For this review, take the finished solid that the model builds, in its own axes (mm). Face numbers are marked on the shaded views. A direction names the side the tool comes from. Round coordinates to 2 decimals unless told otherwise and drop trailing zeros. Write each loop counter-clockwise with the first axis right and the second up, starting at its lowest first coordinate (ties: lowest second). Pieces come first, ordered by that corner, then holes. Notation, with made-up numbers: (60, -24) -> (74, -24) arc R27 ccw to (74, 9) -> close; hole circle Ø8 at (73, -15.5). An arc over 180 degrees is marked (long way). Answer in a Markdown table with one row per item.
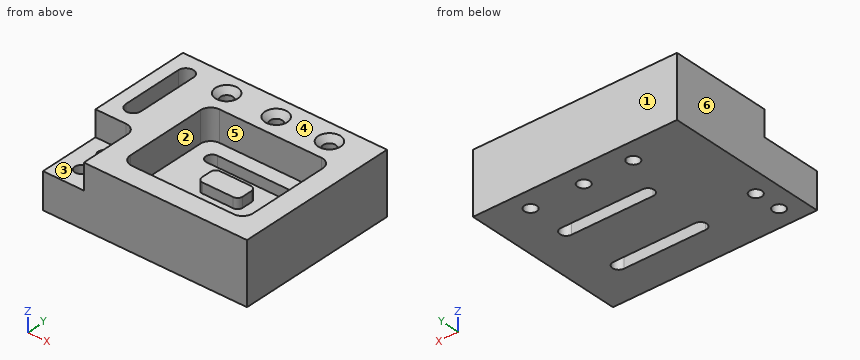
from build123d import *

# Parameters (mm, degrees)
SKETCH1_W           = 200
SKETCH1_H           = 160
BASE_EXTRUDE_DEPTH  = 60
CUT_EXTRUDE1_DEPTH  = 30
CUT_EXTRUDE2_DEPTH  = 25
HOLE1_D             = 12
HOLE1_CSINK_D       = 22
HOLE1_CSINK_ANGLE   = 82
HOLE4_D             = 12
HOLE4_CSINK_D       = 22
HOLE4_CSINK_ANGLE   = 82
HOLE5_D             = 12
HOLE5_CSINK_D       = 22
HOLE5_CSINK_ANGLE   = 82
SKETCH21_R          = 6
CUT_EXTRUDE4_DEPTH  = 133.759180474
CUT_EXTRUDE5_DEPTH  = 25
CUT_EXTRUDE6_DEPTH  = 132.52946438
BOSS_EXTRUDE1_DEPTH = 10


with BuildPart() as part:
    # Sketch1 → Base-Extrude (new body)
    with BuildSketch(Plane.XY):
        Rectangle(SKETCH1_W, SKETCH1_H)
    extrude(amount=-BASE_EXTRUDE_DEPTH)

    # Sketch2 → Cut-Extrude1 (cut)
    with BuildSketch(Plane.XY):
        with BuildLine():
            Line((-30, 40), (70, 40))
            ThreePointArc((70, 40), (77.071067812, 37.071067812), (80, 30))
            Line((80, 30), (80, -50))
            ThreePointArc((80, -50), (77.071067812, -57.071067812), (70, -60))
            Line((70, -60), (-30, -60))
            ThreePointArc((-30, -60), (-37.071067812, -57.071067812), (-40, -50))
            Line((-40, -50), (-40, 30))
            ThreePointArc((-40, 30), (-37.071067812, 37.071067812), (-30, 40))
        make_face()
    extrude(amount=-CUT_EXTRUDE1_DEPTH, mode=Mode.SUBTRACT)

    # Sketch3 → Cut-Extrude2 (cut)
    with BuildSketch(Plane.XY):
        with BuildLine():
            Line((-120, -20), (-70, -20))
            ThreePointArc((-70, -20), (-62.928932188, -22.928932188), (-60, -30))
            Line((-60, -30), (-60, -100))
            Line((-60, -100), (-120, -100))
            Line((-120, -100), (-120, -20))
        make_face()
    extrude(amount=-CUT_EXTRUDE2_DEPTH, mode=Mode.SUBTRACT)

    # Hole1 (through all)
    with Locations(Plane.XY):
        with Locations((-40, 60)):
            CounterSinkHole(HOLE1_D / 2, HOLE1_CSINK_D / 2, counter_sink_angle=HOLE1_CSINK_ANGLE)

    # Hole4 (through all)
    with Locations(Plane(origin=(41.997272993, -0.127725249, 0), x_dir=(1, 0, 0), z_dir=(0, 0, 1))):
        with Locations((-33.333333333, 60)):
            CounterSinkHole(HOLE4_D / 2, HOLE4_CSINK_D / 2, counter_sink_angle=HOLE4_CSINK_ANGLE)

    # Hole5 (through all)
    with Locations(Plane(origin=(100.148393301, 0.657149803, 0), x_dir=(1, 0, 0), z_dir=(0, 0, 1))):
        with Locations((-40, 60)):
            CounterSinkHole(HOLE5_D / 2, HOLE5_CSINK_D / 2, counter_sink_angle=HOLE5_CSINK_ANGLE)

    # Sketch21 → Cut-Extrude4 (cut, through all)
    with BuildSketch(Plane.XY.offset(-25)):
        with Locations((-80, -33.333333333)):
            Circle(SKETCH21_R)
        with Locations((-80, -60)):
            Circle(SKETCH21_R)
    extrude(amount=-CUT_EXTRUDE4_DEPTH, mode=Mode.SUBTRACT)

    # Sketch22 → Cut-Extrude5 (cut)
    with BuildSketch(Plane.XY):
        with BuildLine():
            Line((-72.5, 60), (-72.5, 0))
            ThreePointArc((-72.5, 0), (-80, -7.5), (-87.5, 0))
            Line((-87.5, 0), (-87.5, 60))
            ThreePointArc((-87.5, 60), (-80, 67.5), (-72.5, 60))
        make_face()
    extrude(amount=-CUT_EXTRUDE5_DEPTH, mode=Mode.SUBTRACT)

    # Sketch23 → Cut-Extrude6 (cut, through all)
    with BuildSketch(Plane.XY.offset(-30)):
        with BuildLine():
            Line((-20, 26), (60.148393301, 26))
            ThreePointArc((60.148393301, 26), (66.148393301, 20), (60.148393301, 14))
            Line((60.148393301, 14), (-20, 14))
            ThreePointArc((-20, 14), (-26, 20), (-20, 26))
        make_face()
        with BuildLine():
            Line((-20, -34), (60.148393301, -34))
            ThreePointArc((60.148393301, -34), (66.148393301, -40), (60.148393301, -46))
            Line((60.148393301, -46), (-20, -46))
            ThreePointArc((-20, -46), (-26, -40), (-20, -34))
        make_face()
    extrude(amount=-CUT_EXTRUDE6_DEPTH, mode=Mode.SUBTRACT)

    # Sketch24 → Boss-Extrude1 (add)
    with BuildSketch(Plane.XY.offset(-30)):
        with BuildLine():
            Line((5, 0), (35, 0))
            ThreePointArc((35, 0), (38.535533906, -1.464466094), (40, -5))
            Line((40, -5), (40, -15))
            ThreePointArc((40, -15), (38.535533906, -18.535533906), (35, -20))
            Line((35, -20), (5, -20))
            ThreePointArc((5, -20), (1.464466094, -18.535533906), (0, -15))
            Line((0, -15), (0, -5))
            ThreePointArc((0, -5), (1.464466094, -1.464466094), (5, 0))
        make_face()
    extrude(amount=BOSS_EXTRUDE1_DEPTH)


solid = part.part
1) Clearance check with flat-ended pins moving along their axes: pin 1 Ø1.5 at (x, y) = (36.5, -11) entering from +Z; pin 2 Ø4.5 at (x, y) = (-79, 19.5) entering from +Z. State where each tip first meets the part, or that it passes through.
Solved:
| item | result |
|---|---|
| pin 1 | z = -20 |
| pin 2 | z = -25 |
2) Consider section C-C on z = -46. State the section outline as (x, y) points, then the cut area to 3 significant figures.
Solved:
| item | result |
|---|---|
| outline | (-100, -80) -> (100, -80) -> (100, 80) -> (-100, 80) -> close; hole circle Ø12 at (-80, -60); hole circle Ø12 at (-80, -33.33); hole circle Ø12 at (-40, 60); hole (-20, -46) -> (60.15, -46) arc R6 ccw to (60.15, -34) -> (-20, -34) arc R6 ccw to start; hole (-20, 14) -> (60.15, 14) arc R6 ccw to (60.15, 26) -> (-20, 26) arc R6 ccw to start; hole circle Ø12 at (8.66, 59.87); hole circle Ø12 at (60.15, 60.66) |
| area | 29,300 mm² |
3) For line 1 (Y direction, x = -80, z = -51); line 2 (Y direction, x = -12.5, z = -41.5); line 3 (X direction, y = 60, z = -47), list the stretches that pass through material, from the lowest coordinate up. Write a range as [from, to].
Solved:
| item | result |
|---|---|
| line 1 | [-80, -66], [-54, -39.33], [-27.33, 80] |
| line 2 | [-80, -46], [-34, 14], [26, 80] |
| line 3 | [-100, -46], [-34, 2.67], [14.66, 54.18], [66.11, 100] |
4) Mouldability with a two-part tool opening along X and no side actions: class the marked faces 4, 5 and 6 as pulls with the +X half, pulls with the -X half, needs draft (parallel to the pull), parting line crosses it, or undercut.
Solved:
| item | result |
|---|---|
| face 4 | needs draft |
| face 5 | undercut |
| face 6 | pulls with the -X half |
5) Consider section B-B on y = -42.5. State the section outline as (x, z) points, then the cut area to 3 significant figures.
Solved:
| item | result |
|---|---|
| outline | (-100, -60) -> (-25.45, -60) -> (-25.45, -30) -> (-40, -30) -> (-40, 0) -> (-60, 0) -> (-60, -25) -> (-100, -25) -> close; (65.6, -60) -> (100, -60) -> (100, 0) -> (80, 0) -> (80, -30) -> (65.6, -30) -> close |
| area | 4,670 mm² |
6) Consider section A-A on x = 23. State the section outline as (y, z) points.
Solved:
| item | result |
|---|---|
| outline | (-80, -60) -> (-46, -60) -> (-46, -30) -> (-60, -30) -> (-60, 0) -> (-80, 0) -> close; (-34, -60) -> (14, -60) -> (14, -30) -> (0, -30) -> (0, -20) -> (-20, -20) -> (-20, -30) -> (-34, -30) -> close; (26, -60) -> (80, -60) -> (80, 0) -> (40, 0) -> (40, -30) -> (26, -30) -> close |
7) Consider section D-D on y = -70. State the section outline as (x, z) points, then the cut area to 3 significant figures.
Solved:
| item | result |
|---|---|
| outline | (-100, -60) -> (100, -60) -> (100, 0) -> (-60, 0) -> (-60, -25) -> (-100, -25) -> close |
| area | 11,000 mm² |
8) For the marked faces 1, 2 and 3, list the 3-axis set-ups (+Z, -Z, +X, -X, +Y, -Y) from which the entire face can be reached by the end or side of a thin tool; tool diameter is ignored.
Solved:
| item | result |
|---|---|
| face 1 | +Z, -Z, +X, -X, +Y |
| face 2 | +Z |
| face 3 | +Z, -X, -Y |
